Autodesk Inventor part; units mm, degrees
ref_plane "YZ Plane" through (0, 0, 0) normal (1, 0, 0) x (0, 1, 0)
ref_plane "XZ Plane" through (0, 0, 0) normal (0, 1, 0) x (-1, 0, 0)
ref_plane "XY Plane" through (0, 0, 0) normal (0, 0, 1) x (1, 0, 0)
sketch "Sketch1" plane through (0, 0, 0) normal (1, 0, 0) x (0, 1, 0)
  circle A0 centre (0, 0) radius 4
  dimension "d0" = 8
extrude "Extrusion1" add sketch "Sketch1" along normal blind 0.5
sketch "Sketch2" plane through (0.5, 0, 0) normal (1, 0, 0) x (0, 0, -1)
  circle A0 centre (0, 0) radius 2.9
  circle A1 centre (0, 0) radius 2.75
  line L0 (0, 0) -> (-1.8, 0)
  line L1 (-1.8, 0) -> (-1.8, 3.3564)
  line L2 (-1.8, 3.3564) -> (0, 3.3564)
  line L3 (0, 3.3564) -> (0, 0)
  line L4 (-1.8, 3.3564) -> (1.8, 3.3564)
  line L5 (1.8, 3.3564) -> (1.8, -4.1498)
  line L6 (1.8, -4.1498) -> (-1.8, -4.1498)
  line L7 (-1.8, -4.1498) -> (-1.8, 3.3564)
  dimension "d3" = 5.8
  dimension "d6" = 5.5
  dimension "d7" = 1.8
  dimension "d8" = 3.6
extrude "Extrusion2" add sketch "Sketch2" along normal blind 9.7 contours A0 L5 A1 | L5 A1 L3 A0 | A0 L7 A1 L5 | L3 A1 L1 A0 | L5 A1 L7 L0 L3 | A1 L5 | A0 L1 A1 L7 | L3 L0 L1 A1 | A1 L1 L7
sketch "Sketch3" plane through (10.2, 0, 0) normal (1, 0, 0) x (0, 0, -1)
  circle A0 centre (0, 0) radius 2.75
  line L0 (0, 0) -> (-1.8, 0)
  line L1 (-1.8, 0) -> (-1.8, 4.5353)
  line L2 (-1.8, 4.5353) -> (1.8, 4.5353)
  line L3 (1.8, 4.5353) -> (1.8, -4.8197)
  line L4 (1.8, -4.8197) -> (-1.8, -4.8197)
  line L5 (-1.8, -4.8197) -> (-1.8, 4.5353)
  point P0 (-1.8, -2.0791)
  point P1 (1.8, -2.0791)
  point P2 (1.8, 2.0791)
  point P3 (-1.8, 2.0791)
  dimension "d9" = 5.5
  dimension "d10" = 1.8
  dimension "d11" = 3.6
extrude "Extrusion3" add sketch "Sketch3" along normal blind 27 contours L3 A0 L5 L1
properties part number "wielas"
The listing builds one solid part. Answer for the finished solid, in the listing's coordinates (mm). A direction names the side the tool comes from. Give positions to 0.01 mm unless a question says otherwise; leave off trailing zeros. Loops run counter-clockwise (first coordinate to the right, second up) from the corner with the lowest first, then second, coordinate; pieces in that order, holes last. Notation, with made-up numbers: M -25,75.25 L 31,75.25 A13 ccw 31,82.25 Z; hole C 77,-4.5 d10. An arc over 180 degrees is marked long. Answer as CSV lines item,"result".
Item 1: The part is cut by section A-A (y = 0). Give the vertices of the cut face in (x, z), and give its area (3 significant figures).
Values follow:
outline,"M 0,-4 L 0.5,-4 L 0.5,-2.9 L 10.2,-2.9 L 10.2,-1.8 L 37.2,-1.8 L 37.2,1.8 L 10.2,1.8 L 10.2,2.9 L 0.5,2.9 L 0.5,4 L 0,4 Z"
area,"157 mm^2"
Item 2: The part is cut by section C-C (x = 14.5). Give the vertices of the cut face in (y, z), and give its area (3 significant figures).
Values follow:
outline,"M -2.08,-1.8 L 2.08,-1.8 A2.75 ccw 2.08,1.8 L -2.08,1.8 A2.75 ccw Z"
area,"18.3 mm^2"
Item 3: Which of the six approach directions +Z, -Z, +X, -X, +Y, -Y give full straight-line access (tool end or side, diameter ignored) to faces 1 (the cylindrical face through (23.51, -2.75, -0.03)), 2 (the flat face through (0.5, 3, 1)), 3 (the flat face through (24, 0, -1.8)), 4 (the cylindrical face through (23.51, 2.75, 0.03)), 5 (the flat face through (24, 0, 1.8))?
Values follow:
face 1,"+X, -Y"
face 2,"+X"
face 3,"-Z, +X, +Y, -Y"
face 4,"+X, +Y"
face 5,"+Z, +X, +Y, -Y"
Item 4: The part is cut by section D-D (x = 7). Give the vertices of the cut face in (y, z), and give its area (3 significant figures).
Values follow:
outline,"C 0,0 d5.8"
area,"26.4 mm^2"
Item 5: The part is cut by section B-B (z = 0). Give the vertices of the cut face in (x, y), and give its area (3 significant figures).
Values follow:
outline,"M 0,-4 L 0.5,-4 L 0.5,-2.9 L 10.2,-2.9 L 10.2,-2.75 L 37.2,-2.75 L 37.2,2.75 L 10.2,2.75 L 10.2,2.9 L 0.5,2.9 L 0.5,4 L 0,4 Z"
area,"209 mm^2"
Item 6: Straight lines are drawn through the part: line 1 along X through (y, z) = (-2.75, 1.5); line 2 along Z through (x, y) = (20, 0.5); line 3 along X through (y, z) = (0.5, -2.5). For each, find the intervals that lie inside material, in ascending order. Write a range as [from, to].
Values follow:
line 1,"x = [0, 0.5]"
line 2,"z = [-1.8, 1.8]"
line 3,"x = [0, 10.2]"
Item 7: Given pin 1 Ø1 at (x, z) = (18, 1.5) entering from +Y; pin 2 Ø3 at (x, y) = (8, 1) entering from -Z; pin 3 Ø3 at (x, y) = (12.5, -1.5) entering from -Z, each flat-ended and moving along its own axis, determine where each tip first touches the part or whether it passes through.
Values follow:
pin 1,"stops at y = 2.56"
pin 2,"stops at z = -2.9"
pin 3,"stops at z = -1.8"
